```python
from build123d import *

# Parameters (mm, degrees)
F0_R     = 2.5
F1_DEPTH = 2


# Not quite as in the source:
# - a feature names something its author has since deleted; it is built from what else it names


with BuildPart() as f1:
    # F0 (on Top) → F1 (new body)
    with BuildSketch(Plane.XY):
        with BuildLine():
            ThreePointArc((40, 15), (38.5355339059, 18.5355339059), (35, 20))
            Line((35, 20), (-15, 20))
            ThreePointArc((-15, 20), (-18.5355339059, 18.5355339059), (-20, 15))
            Line((-20, 15), (-20, -35))
            ThreePointArc((-20, -35), (-18.5355339059, -38.5355339059), (-15, -40))
            Line((-15, -40), (35, -40))
            ThreePointArc((35, -40), (38.5355339059, -38.5355339059), (40, -35))
            Line((40, -35), (40, 15))
        make_face()
        with Locations((-15, -15)):
            Circle(F0_R, mode=Mode.SUBTRACT)
        with Locations((15, -15)):
            Circle(F0_R, mode=Mode.SUBTRACT)
        with Locations((-15, 15)):
            Circle(F0_R, mode=Mode.SUBTRACT)
        with Locations((15, 15)):
            Circle(F0_R, mode=Mode.SUBTRACT)
    extrude(amount=F1_DEPTH)


solid = f1.part
```
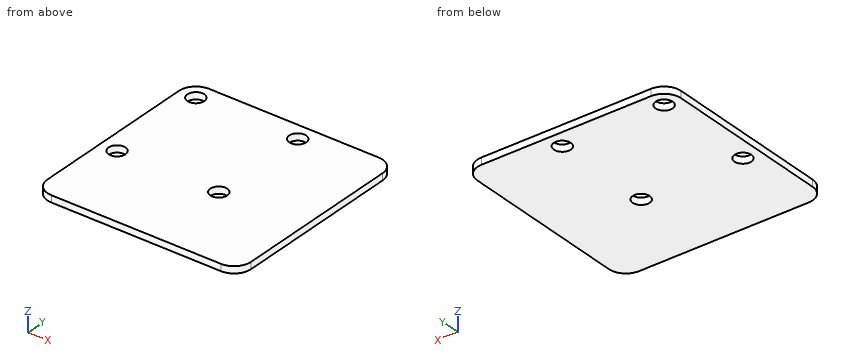
For this review, take the finished solid that the model builds, in its own axes (mm). Round coordinates to 2 decimals unless told otherwise and drop trailing zeros. Write each loop counter-clockwise with the first axis right and the second up, starting at its lowest first coordinate (ties: lowest second). Pieces come first, ordered by that corner, then holes. Notation, with made-up numbers: (0.5, 70) - (25.5, 70) arc R4 cw to (25.5, 76) - close; hole circle Ø5 at (-18.5, 78). An arc over 180 degrees is marked (long way). Put each result on its own line as item: value.
Q1. Insertion check: pin 1 Ø4 at (x, y) = (15, 15) entering from +Z. The pin has a flat end and moves straight along its axis. Give the tip position at first contact, or say it passes through.
Solved:
pin 1: passes through
Q2. Wall thickness on probe 1 along Y at (x, z) = (-15, 1.15): over which ranges is the line inside the solid? List them lowest first.
Solved:
probe 1: y = -40 to -17.5, -12.5 to 12.5, 17.5 to 20
Q3. We need section B-B (x = 15). Give the boundary of the cut face in (y, z), and give its area (3 significant figures).
Solved:
outline: (-40, 0) - (-17.5, 0) - (-17.5, 2) - (-40, 2) - close; (-12.5, 0) - (12.5, 0) - (12.5, 2) - (-12.5, 2) - close; (17.5, 0) - (20, 0) - (20, 2) - (17.5, 2) - close
area: 100 mm2
Q4. We need section A-A (y = -15). Give the boundary of the cut face in (x, z), and give its area (3 significant figures).
Solved:
outline: (-20, 0) - (-17.5, 0) - (-17.5, 2) - (-20, 2) - close; (-12.5, 0) - (12.5, 0) - (12.5, 2) - (-12.5, 2) - close; (17.5, 0) - (40, 0) - (40, 2) - (17.5, 2) - close
area: 100 mm2
